Autodesk Inventor part; units mm, degrees
ref_plane "YZ Plane" through (0, 0, 0) normal (1, 0, 0) x (0, 1, 0)
ref_plane "XZ Plane" through (0, 0, 0) normal (0, 1, 0) x (-1, 0, 0)
ref_plane "XY Plane" through (0, 0, 0) normal (0, 0, 1) x (1, 0, 0)
sketch "Sketch1" plane through (0, 0, 0) normal (0, 1, 0) x (-1, 0, 0)
  line L0 (-250, 125) -> (250, 125)
  line L1 (250, 125) -> (250, -125)
  line L2 (250, -125) -> (-250, -125)
  line L3 (-250, -125) -> (-250, 125)
  line L4 (-250, 125) -> (250, -125) construction
  line L5 (250, 125) -> (-250, -125) construction
  point P0 (0, 0)
  dimension "d0" = 500
  dimension "d1" = 250
extrude "Extrusion1" add sketch "Sketch1" along normal blind 3
sketch "Sketch3" plane through (0, 3, 0) normal (0, 1, 0) x (1, 0, 0)
  line L0 (55.5, 115.125) -> (4.5, 115.125)
  line L1 (4.5, 115.125) -> (4.5, 111.875)
  line L2 (4.5, 111.875) -> (55.5, 111.875)
  line L3 (55.5, 111.875) -> (55.5, 115.125)
  line L4 (55.5, 115.125) -> (4.5, 111.875) construction
  line L5 (4.5, 115.125) -> (55.5, 111.875) construction
  line L6 (-4.5, 115.125) -> (-55.5, 115.125)
  line L7 (-55.5, 115.125) -> (-55.5, 111.875)
  line L8 (-55.5, 111.875) -> (-4.5, 111.875)
  line L9 (-4.5, 111.875) -> (-4.5, 115.125)
  line L10 (-4.5, 115.125) -> (-55.5, 111.875) construction
  line L11 (-55.5, 115.125) -> (-4.5, 111.875) construction
  line L12 (250, 125) -> (-250, 125)
  line L13 (231, 115.125) -> (180, 115.125)
  line L14 (180, 115.125) -> (180, 111.875)
  line L15 (180, 111.875) -> (231, 111.875)
  line L16 (231, 111.875) -> (231, 115.125)
  line L17 (231, 115.125) -> (180, 111.875) construction
  line L18 (180, 115.125) -> (231, 111.875) construction
  line L19 (4.5, 115.125) -> (-4.5, 115.125)
  line L20 (-4.5, 115.125) -> (-4.5, 111.875)
  line L21 (-4.5, 111.875) -> (4.5, 111.875)
  line L22 (4.5, 111.875) -> (4.5, 115.125)
  line L23 (-180, 115.125) -> (-231, 115.125)
  line L24 (-231, 115.125) -> (-231, 111.875)
  line L25 (-231, 111.875) -> (-180, 111.875)
  line L26 (-180, 111.875) -> (-180, 115.125)
  line L27 (250, 125) -> (250, -125)
  line L28 (55.5, 103.625) -> (4.5, 103.625)
  line L29 (4.5, 103.625) -> (4.5, 100.375)
  line L30 (4.5, 100.375) -> (55.5, 100.375)
  line L31 (55.5, 100.375) -> (55.5, 103.625)
  line L32 (55.5, 103.625) -> (4.5, 100.375) construction
  line L33 (4.5, 103.625) -> (55.5, 100.375) construction
  line L34 (-4.5, 103.625) -> (-55.5, 103.625)
  line L35 (-55.5, 103.625) -> (-55.5, 100.375)
  line L36 (-55.5, 100.375) -> (-4.5, 100.375)
  line L37 (-4.5, 100.375) -> (-4.5, 103.625)
  line L38 (-4.5, 103.625) -> (-55.5, 100.375) construction
  line L39 (-55.5, 103.625) -> (-4.5, 100.375) construction
  line L40 (4.5, 103.625) -> (-4.5, 103.625)
  line L41 (-4.5, 103.625) -> (-4.5, 100.375)
  line L42 (-4.5, 100.375) -> (4.5, 100.375)
  line L43 (4.5, 100.375) -> (4.5, 103.625)
  line L44 (-180, 103.625) -> (-231, 103.625)
  line L45 (-231, 103.625) -> (-231, 100.375)
  line L46 (-231, 100.375) -> (-180, 100.375)
  line L47 (-180, 100.375) -> (-180, 103.625)
  line L48 (250, 113.5) -> (250, -136.5)
  line L49 (253.2147, 0) -> (-252.6779, 0)
  line L50 (231, 103.625) -> (180, 103.625)
  line L51 (180, 103.625) -> (180, 100.375)
  line L52 (180, 100.375) -> (231, 100.375)
  line L53 (231, 100.375) -> (231, 103.625)
  line L54 (231, 103.625) -> (180, 100.375) construction
  line L55 (180, 103.625) -> (231, 100.375) construction
  line L56 (55.5, -115.125) -> (4.5, -115.125)
  line L57 (4.5, -115.125) -> (4.5, -111.875)
  line L58 (4.5, -111.875) -> (55.5, -111.875)
  line L59 (55.5, -111.875) -> (55.5, -115.125)
  line L60 (55.5, -115.125) -> (4.5, -111.875) construction
  line L61 (4.5, -115.125) -> (55.5, -111.875) construction
  line L62 (-4.5, -115.125) -> (-55.5, -115.125)
  line L63 (-55.5, -115.125) -> (-55.5, -111.875)
  line L64 (-55.5, -111.875) -> (-4.5, -111.875)
  line L65 (-4.5, -111.875) -> (-4.5, -115.125)
  line L66 (-4.5, -115.125) -> (-55.5, -111.875) construction
  line L67 (-55.5, -115.125) -> (-4.5, -111.875) construction
  line L68 (250, -125) -> (-250, -125)
  line L69 (231, -115.125) -> (180, -115.125)
  line L70 (180, -115.125) -> (180, -111.875)
  line L71 (180, -111.875) -> (231, -111.875)
  line L72 (231, -111.875) -> (231, -115.125)
  line L73 (231, -115.125) -> (180, -111.875) construction
  line L74 (180, -115.125) -> (231, -111.875) construction
  line L75 (4.5, -115.125) -> (-4.5, -115.125)
  line L76 (-4.5, -115.125) -> (-4.5, -111.875)
  line L77 (-4.5, -111.875) -> (4.5, -111.875)
  line L78 (4.5, -111.875) -> (4.5, -115.125)
  line L79 (-180, -115.125) -> (-231, -115.125)
  line L80 (-231, -115.125) -> (-231, -111.875)
  line L81 (-231, -111.875) -> (-180, -111.875)
  line L82 (-180, -111.875) -> (-180, -115.125)
  line L83 (4.5, -103.625) -> (-4.5, -103.625)
  line L84 (-4.5, -100.375) -> (4.5, -100.375)
  line L85 (-4.5, -100.375) -> (-4.5, -103.625)
  line L86 (-4.5, -103.625) -> (-4.5, -100.375)
  line L87 (-55.5, -100.375) -> (-4.5, -100.375)
  line L88 (-55.5, -103.625) -> (-55.5, -100.375)
  line L89 (-4.5, -103.625) -> (-55.5, -100.375) construction
  line L90 (-55.5, -103.625) -> (-4.5, -100.375) construction
  line L91 (-4.5, -103.625) -> (-55.5, -103.625)
  line L92 (4.5, -103.625) -> (4.5, -100.375)
  line L93 (4.5, -100.375) -> (4.5, -103.625)
  line L94 (55.5, -103.625) -> (4.5, -103.625)
  line L95 (4.5, -100.375) -> (55.5, -100.375)
  line L96 (55.5, -103.625) -> (4.5, -100.375) construction
  line L97 (4.5, -103.625) -> (55.5, -100.375) construction
  line L98 (55.5, -100.375) -> (55.5, -103.625)
  line L99 (-180, -100.375) -> (-180, -103.625)
  line L100 (-180, -103.625) -> (-231, -103.625)
  line L101 (-231, -100.375) -> (-180, -100.375)
  line L102 (-231, -103.625) -> (-231, -100.375)
  line L103 (180, -103.625) -> (180, -100.375)
  line L104 (231, -103.625) -> (180, -103.625)
  line L105 (180, -100.375) -> (231, -100.375)
  line L106 (231, -103.625) -> (180, -100.375) construction
  line L107 (180, -103.625) -> (231, -100.375) construction
  line L108 (231, -100.375) -> (231, -103.625)
  point P0 (0, 0)
  point P1 (30, 113.5)
  point P2 (-30, 113.5)
  point P3 (205.5, 113.5)
  point P4 (0, -11.5)
  point P5 (30, 102)
  point P6 (-30, 102)
  point P7 (-250, 113.5)
  point P8 (205.5, 102)
  point P9 (30, -113.5)
  point P10 (-30, -113.5)
  point P11 (205.5, -113.5)
  point P12 (250, -113.5)
  point P13 (-250, -113.5)
  point P14 (-30, -102)
  point P15 (30, -102)
  point P16 (205.5, -102)
  dimension "d28" = 51
  dimension "d29" = 3.25
  dimension "d30" = 51
  dimension "d31" = 3.25
  dimension "d32" = 4.5
  dimension "d33" = 9
  dimension "d34" = 9.875
  dimension "d35" = 9.875
  dimension "d36" = 51
  dimension "d37" = 3.25
  dimension "d38" = 124.5
  dimension "d39" = 9.875
  dimension "d40" = 51
  dimension "d41" = 3.25
  dimension "d42" = 124.5
  dimension "d43" = 9.875
  dimension "d46" = 11.5
  dimension "d53" = 11.5
extrude "Extrusion3" cut sketch "Sketch3" against normal blind 10
properties part number "plaat"
The listing builds one solid part. Answer for the finished solid, in the listing's coordinates (mm). Coordinates: 2 decimals unless noted, no trailing zeros. Loops run counter-clockwise (first coordinate to the right, second up) from the corner with the lowest first, then second, coordinate; pieces in that order, holes last. Notation, with made-up numbers: (-23, -31) -> (-11, -31) arc R19 cw to (-11, -15) -> close; hole circle Ø11 at (62.5, 42.5). An arc over 180 degrees is marked (long way). Return JSON: item names as keys, results as strings. Group by question number.
(1) Find the intervals of material crossed by probe 1 along Z at (x, y) = (-220, 1.9) (3 decimals); probe 2 along X at (y, z) = (0.2, 101), in increasing order. Write a range as from..to.
(2) A cutting plane is placed at A-A on x = -38.5. Write down the section's boundary in (y, z) (3 decimals).
(3) A cutting plane is placed at B-B on y = 0.85. Count the separate pieces of the cut face and the enclosed holes in it, and give its area (3 significant figures).
The answers:
{
 "1": {"probe 1": "z = -125..-115.125, -111.875..-103.625, -100.375..100.375, 103.625..111.875, 115.125..125", "probe 2": "x = -250..-231, -180..-55.5, 55.5..180, 231..250"},
 "2": {"outline": "(0, -125) -> (3, -125) -> (3, -115.125) -> (0, -115.125) -> close; (0, -111.875) -> (3, -111.875) -> (3, -103.625) -> (0, -103.625) -> close; (0, -100.375) -> (3, -100.375) -> (3, 100.375) -> (0, 100.375) -> close; (0, 103.625) -> (3, 103.625) -> (3, 111.875) -> (0, 111.875) -> close; (0, 115.125) -> (3, 115.125) -> (3, 125) -> (0, 125) -> close"},
 "3": {"separate pieces": "1", "enclosed holes": "12", "area": "122,000 mm^2"}
}
